The model under review builds one solid part; all positions refer to its coordinate system, in mm. Face numbers are marked on the shaded views. Coordinates: 2 decimals unless noted, no trailing zeros. Order: outer loops, then holes, each group sorted by start corner. A loop starts at its lowest first (then second) coordinate and runs counter-clockwise, first axis right, second up.
from build123d import *

# Parameters (mm, degrees)
SKETCH1_R           = 22.098
SKETCH1_R_2         = 9.525
BOSS_EXTRUDE1_DEPTH = 5.08
SKETCH4_R           = 1.4605
SKETCH4_R_2         = 1.524
CUT_EXTRUDE1_DEPTH  = 58.42
SKETCH5_R           = 12.7
CUT_EXTRUDE2_DEPTH  = 29.21
SKETCH5_3_R         = 12.7
BOSS_EXTRUDE2_DEPTH = 101.6
SKETCH6_R           = 7.62
CUT_EXTRUDE3_DEPTH  = 17.78
SKETCH7_W           = 15.24
SKETCH7_H           = 11.096968574
CUT_EXTRUDE4_DEPTH  = 107.297710267


with BuildPart() as part:
    # Sketch1 → Boss-Extrude1 (new body)
    # profile 1 of 2: a face of its own
    with BuildSketch(Plane(origin=(0, 0, 0), x_dir=(1, 0, 0), z_dir=(0, 1, 0))):
        with Locations(Location((0, 0, 0), (0, 0, 270))):
            Circle(SKETCH1_R)
        Circle(SKETCH1_R_2, mode=Mode.SUBTRACT)
    # profile 2 of 2: a face of its own
    with BuildSketch(Plane(origin=(0, 0, 0), x_dir=(1, 0, 0), z_dir=(0, 1, 0))):
        Circle(SKETCH1_R_2)
    extrude(amount=BOSS_EXTRUDE1_DEPTH)

    # Sketch4 → Cut-Extrude1 (cut)
    with BuildSketch(Plane(origin=(0, 5.08, 0), x_dir=(1, 0, 0), z_dir=(0, 1, 0))):
        with Locations(Location((13.96833752, 12.106825614, 0), (0, 0, 270))):
            Circle(SKETCH4_R)
        with Locations(Location((13.96833752, -12.106825614, 0), (0, 0, 270))):
            Circle(SKETCH4_R)
        with Locations(Location((-18.48485, 0, 0), (0, 0, 270))):
            Circle(SKETCH4_R_2)
    extrude(amount=-CUT_EXTRUDE1_DEPTH, mode=Mode.SUBTRACT)

    # Sketch5 → Cut-Extrude2 (cut)
    with BuildSketch(Plane.XZ):
        with Locations(Location((0, 0, 0), (0, 0, 270))):
            Circle(SKETCH5_R)
    extrude(amount=-CUT_EXTRUDE2_DEPTH, mode=Mode.SUBTRACT)

    # Sketch5_3 → Boss-Extrude2 (add)
    with BuildSketch(Plane.XZ):
        with Locations(Location((0, 0, 0), (0, 0, 270))):
            Circle(SKETCH5_3_R)
    extrude(amount=-BOSS_EXTRUDE2_DEPTH)

    # Sketch6 → Cut-Extrude3 (cut)
    with BuildSketch(Plane.XZ):
        with Locations(Location((0, 0, 0), (0, 0, 270))):
            Circle(SKETCH6_R)
    extrude(amount=-CUT_EXTRUDE3_DEPTH, mode=Mode.SUBTRACT)

    # Sketch7 → Cut-Extrude4 (cut, through all)
    with BuildSketch(Plane(origin=(0, 0, 0), x_dir=(0, 0, -1), z_dir=(1, 0, 0))):
        with Locations((0, 10.628484287)):
            Rectangle(SKETCH7_W, SKETCH7_H)
    extrude(amount=-CUT_EXTRUDE4_DEPTH, mode=Mode.SUBTRACT)


solid = part.part
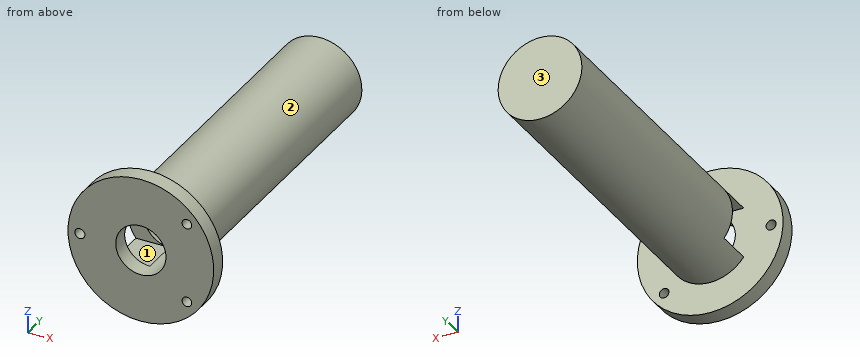
(1) Consider section B-B (x = 1.5). Give the boundary of the cut face in (y, z), then the cut area to 3 significant figures.
(2) The part is to be moulded in two halves that separate along Z. For the marked faces 1, 2 and 3, say which applies: +Z half, -Z half, draft (parallel to the pull), parting line (faces both ways), or undercut.
(3) Insertion check: pin 1 Ø3.5 at (x, z) = (13.97, 12.11) entering from +Y; pin 2 Ø9 at (x, z) = (0, 0) entering from -Y; pin 3 Ø10 at (x, y) = (5.5, 31) entering from +Z. Each pin has a flat end and moves straight along its axis. Give the tip position at first contact, or say it passes through.
(4) Consider section A-A (z = 0). Give the boundary of the cut face in (x, y), then the cut area to 3 significant figures.
(5) Wall thickness on line 1 (X direction, y = 2.25, z = 0); line 2 (Y direction, x = 15, z = 8.5); line 3 (Y direction, x = 4, z = -5.5): over which ranges is each line inside the solid? List them lowest first.
(6) Consider section C-C (y = 76). Give the boundary of the cut face in (x, z), then the cut area to 3 significant figures.
(7) Consider section D-D (z = 6.5). Give the boundary of the cut face in (x, y), then the cut area to 3 significant figures.
Findings:
1. outline: (0, -22.05) - (5.08, -22.05) - (5.08, -12.61) - (101.6, -12.61) - (101.6, 12.61) - (5.08, 12.61) - (5.08, 22.05) - (0, 22.05) - (0, 7.47) - (17.78, 7.47) - (17.78, -7.47) - (0, -7.47) - close
1. area: 2,390 mm2
2. face 1: undercut
2. face 2: parting line
2. face 3: draft
3. pin 1: stops at y = 5.08
3. pin 2: stops at y = 17.78
3. pin 3: stops at z = 12.69
4. outline: (-22.1, 0) - (-20.01, 0) - (-20.01, 5.08) - (-22.1, 5.08) - close; (-16.96, 0) - (-7.62, 0) - (-7.62, 5.08) - (-16.96, 5.08) - close; (-12.7, 16.18) - (-7.62, 16.18) - (-7.62, 17.78) - (7.62, 17.78) - (7.62, 0) - (22.1, 0) - (22.1, 5.08) - (12.7, 5.08) - (12.7, 101.6) - (-12.7, 101.6) - close
4. area: 2,330 mm2
5. line 1: x = -22.1 to -20.01, -16.96 to -7.62, 7.62 to 22.1
5. line 2: y = 0 to 5.08
5. line 3: y = 17.78 to 101.6
6. outline: circle Ø25.4 at (0, 0)
6. area: 507 mm2
7. outline: (-21.12, 0) - (-3.98, 0) - (-3.98, 5.08) - (-21.12, 5.08) - close; (-10.91, 16.18) - (-3.98, 16.18) - (-3.98, 17.78) - (3.98, 17.78) - (3.98, 0) - (21.12, 0) - (21.12, 5.08) - (10.91, 5.08) - (10.91, 101.6) - (-10.91, 101.6) - close
7. area: 2,100 mm2
